Part model, mm, in its own coordinate system. A direction names the side the tool comes from. Give positions to 0.01 mm unless a question says otherwise; leave off trailing zeros. Loops run counter-clockwise (first coordinate to the right, second up) from the corner with the lowest first, then second, coordinate; pieces in that order, holes last. Notation, with made-up numbers: M 55,-34 L 69,-34 A31 ccw 69,5 Z; hole C 1.25,76 d7. An arc over 180 degrees is marked long. Answer in a Markdown table with one row per item.
from build123d import *

# Parameters (mm, degrees)
ESQUISSE1_W              = 130
ESQUISSE1_H              = 167
BOSS_EXTRU_1_DEPTH       = 3
ESQUISSE6_R              = 3.5
ESQUISSE6_R_2            = 4
BOSS_EXTRU_3_DEPTH       = 5
ESQUISSE11_W             = 67
ESQUISSE11_H             = 10
BOSS_EXTRU_6_DEPTH       = 49
ENL_V_MAT_EXTRU_3_REACH  = 113.374
ESQUISSE12_R             = 7.5
ESQUISSE12_W             = 7
ESQUISSE12_H             = 10
ESQUISSE13_R             = 9.4
ENL_V_MAT_EXTRU_4_DEPTH  = 65.5
BOSS_EXTRU_7_DEPTH       = 1.5
ESQUISSE15_W             = 20
ESQUISSE15_H             = 4
ENL_V_MAT_EXTRU_5_DEPTH  = 43.7
ESQUISSE16_W             = 21
ESQUISSE16_H             = 10
BOSS_EXTRU_8_DEPTH       = 78.5
ESQUISSE17_W             = 10.5
ESQUISSE17_H             = 10
ESQUISSE17_W_2           = 20
ESQUISSE17_H_2           = 4
ENL_V_MAT_EXTRU_6_DEPTH  = 24.2
ENL_V_MAT_EXTRU_7_REACH  = 148.361
ESQUISSE18_R             = 7.5
ESQUISSE19_R             = 9.4
ENL_V_MAT_EXTRU_8_DEPTH  = 65.5
BOSS_EXTRU_9_DEPTH       = 1.5
ESQUISSE21_R             = 2.3
ESQUISSE21_R_2           = 1.8
ENL_V_MAT_EXTRU_9_DEPTH  = 6.1
ESQUISSE22_R             = 1.7
ENL_V_MAT_EXTRU_10_DEPTH = 107.288522428


with BuildPart() as part:
    # Esquisse1 → Boss.-Extru.1 (new body)
    with BuildSketch(Plane(origin=(0, 0, 0), x_dir=(1, 0, 0), z_dir=(0, 1, 0))):
        Rectangle(ESQUISSE1_W, ESQUISSE1_H)
    extrude(amount=BOSS_EXTRU_1_DEPTH)

    # Esquisse6 → Boss.-Extru.3 (add)
    with BuildSketch(Plane(origin=(0, 3, 0), x_dir=(1, 0, 0), z_dir=(0, 1, 0))):
        with Locations(Location((-8, -73.5, 0), (0, 0, 90))):
            Circle(ESQUISSE6_R)
        with Locations(Location((-8, -50.5, 0), (0, 0, 90))):
            Circle(ESQUISSE6_R)
        with Locations(Location((50, -50.5, 0), (0, 0, 90))):
            Circle(ESQUISSE6_R)
        with Locations(Location((50, -73.5, 0), (0, 0, 90))):
            Circle(ESQUISSE6_R)
        with Locations(Location((56, 43.5, 0), (0, 0, 90))):
            Circle(ESQUISSE6_R_2)
        with Locations(Location((56, -34.732, 0), (0, 0, 90))):
            Circle(ESQUISSE6_R_2)
        with Locations(Location((-3.436, -35.232, 0), (0, 0, 90))):
            Circle(ESQUISSE6_R_2)
    extrude(amount=BOSS_EXTRU_3_DEPTH)

    # Esquisse11 → Boss.-Extru.6 (add)
    with BuildSketch(Plane.ZY.offset(65)):
        with Locations((-27.5, 8)):
            Rectangle(ESQUISSE11_W, ESQUISSE11_H)
    extrude(amount=-BOSS_EXTRU_6_DEPTH)

    # Esquisse12 → Enlèv. mat.-Extru.3 (cut, up to next)
    with BuildSketch(Plane.XY.offset(6), mode=Mode.PRIVATE) as enl_v_mat_extru_3_sk1:
        with Locations((-47.2, 13)):
            Circle(ESQUISSE12_R)
    enl_v_mat_extru_3_tool1 = extrude(enl_v_mat_extru_3_sk1.sketch, amount=-ENL_V_MAT_EXTRU_3_REACH, mode=Mode.PRIVATE) & part.part
    # Esquisse12 → Enlèv. mat.-Extru.3 (cut, up to next)
    with BuildSketch(Plane.XY.offset(6), mode=Mode.PRIVATE) as enl_v_mat_extru_3_sk2:
        with Locations((-26.8, 13)):
            Circle(ESQUISSE12_R)
    enl_v_mat_extru_3_tool2 = extrude(enl_v_mat_extru_3_sk2.sketch, amount=-ENL_V_MAT_EXTRU_3_REACH, mode=Mode.PRIVATE) & part.part
    # Esquisse12 → Enlèv. mat.-Extru.3 (cut, up to next)
    with BuildSketch(Plane.XY.offset(6), mode=Mode.PRIVATE) as enl_v_mat_extru_3_sk3:
        with Locations((-61.5, 8)):
            Rectangle(ESQUISSE12_W, ESQUISSE12_H)
    enl_v_mat_extru_3_tool3 = extrude(enl_v_mat_extru_3_sk3.sketch, amount=-ENL_V_MAT_EXTRU_3_REACH, mode=Mode.PRIVATE) & part.part
    add(enl_v_mat_extru_3_tool1.solids().sort_by_distance((-47.2, 13, 6))[0], mode=Mode.SUBTRACT)
    add(enl_v_mat_extru_3_tool2.solids().sort_by_distance((-26.8, 13, 6))[0], mode=Mode.SUBTRACT)
    add(enl_v_mat_extru_3_tool3.solids().sort_by_distance((-61.5, 8, 6))[0], mode=Mode.SUBTRACT)

    # Esquisse13 → Enlèv. mat.-Extru.4 (cut)
    with BuildSketch(Plane.XY.offset(6)):
        with Locations((-47.2, 13)):
            Circle(ESQUISSE13_R)
        with Locations((-26.8, 13)):
            Circle(ESQUISSE13_R)
    extrude(amount=-ENL_V_MAT_EXTRU_4_DEPTH, mode=Mode.SUBTRACT)

    # Esquisse14 → Boss.-Extru.7 (add)
    with BuildSketch(Plane.XY.offset(6)):
        with BuildLine():
            Line((-58, 13), (-54.7, 13))
            ThreePointArc((-54.7, 13), (-47.2, 5.5), (-39.7, 13))
            Line((-39.7, 13), (-34.3, 13))
            ThreePointArc((-34.3, 13), (-26.8, 5.5), (-19.3, 13))
            Line((-19.3, 13), (-16, 13))
            Line((-16, 13), (-16, 3))
            Line((-16, 3), (-58, 3))
            Line((-58, 3), (-58, 13))
        make_face()
    extrude(amount=-BOSS_EXTRU_7_DEPTH)

    # Esquisse15 → Enlèv. mat.-Extru.5 (cut)
    with BuildSketch(Plane.ZY.offset(58)):
        with Locations((-28, 11)):
            Rectangle(ESQUISSE15_W, ESQUISSE15_H)
    extrude(amount=-ENL_V_MAT_EXTRU_5_DEPTH, mode=Mode.SUBTRACT)

    # Esquisse16 → Boss.-Extru.8 (add)
    with BuildSketch(Plane(origin=(65, 0, 0), x_dir=(0, 0, -1), z_dir=(1, 0, 0))):
        with Locations((69.6, 8)):
            Rectangle(ESQUISSE16_W, ESQUISSE16_H)
    extrude(amount=-BOSS_EXTRU_8_DEPTH)

    # Esquisse17 → Enlèv. mat.-Extru.6 (cut)
    with BuildSketch(Plane(origin=(0, 0, -80.1), x_dir=(-1, 0, 0), z_dir=(0, 0, -1))):
        with Locations((-59.75, 8)):
            Rectangle(ESQUISSE17_W, ESQUISSE17_H)
        with Locations((-20.5, 11)):
            Rectangle(ESQUISSE17_W_2, ESQUISSE17_H_2)
    extrude(amount=-ENL_V_MAT_EXTRU_6_DEPTH, mode=Mode.SUBTRACT)

    # Esquisse18 → Enlèv. mat.-Extru.7 (cut, up to next)
    with BuildSketch(Plane(origin=(54.5, 0, 0), x_dir=(0, 0, -1), z_dir=(1, 0, 0)), mode=Mode.PRIVATE) as enl_v_mat_extru_7_sk1:
        with Locations((69.6, 13)):
            Circle(ESQUISSE18_R)
    enl_v_mat_extru_7_tool1 = extrude(enl_v_mat_extru_7_sk1.sketch, amount=-ENL_V_MAT_EXTRU_7_REACH, mode=Mode.PRIVATE) & part.part
    add(enl_v_mat_extru_7_tool1.solids().sort_by_distance((54.5, 13, -69.6))[0], mode=Mode.SUBTRACT)

    # Esquisse19 → Enlèv. mat.-Extru.8 (cut)
    with BuildSketch(Plane(origin=(54.5, 0, 0), x_dir=(0, 0, -1), z_dir=(1, 0, 0))):
        with Locations((69.6, 13)):
            Circle(ESQUISSE19_R)
    extrude(amount=-ENL_V_MAT_EXTRU_8_DEPTH, mode=Mode.SUBTRACT)

    # Esquisse20 → Boss.-Extru.9 (add)
    with BuildSketch(Plane(origin=(54.5, 0, 0), x_dir=(0, 0, -1), z_dir=(1, 0, 0))):
        with BuildLine():
            Line((59.1, 13), (62.1, 13))
            ThreePointArc((62.1, 13), (69.6, 5.5), (77.1, 13))
            Line((77.1, 13), (80.1, 13))
            Line((80.1, 13), (80.1, 3))
            Line((80.1, 3), (59.1, 3))
            Line((59.1, 3), (59.1, 13))
        make_face()
    extrude(amount=-BOSS_EXTRU_9_DEPTH)

    # Esquisse21 → Enlèv. mat.-Extru.9 (cut)
    with BuildSketch(Plane(origin=(0, 8, 0), x_dir=(1, 0, 0), z_dir=(0, 1, 0))):
        with Locations(Location((56, 43.5, 0), (0, 0, 270))):
            Circle(ESQUISSE21_R)
        with Locations(Location((56, -34.732, 0), (0, 0, 270))):
            Circle(ESQUISSE21_R)
        with Locations(Location((-3.436, -35.232, 0), (0, 0, 270))):
            Circle(ESQUISSE21_R)
        with Locations(Location((50, -50.5, 0), (0, 0, 270))):
            Circle(ESQUISSE21_R_2)
        with Locations(Location((50, -73.5, 0), (0, 0, 270))):
            Circle(ESQUISSE21_R_2)
        with Locations(Location((-8, -50.5, 0), (0, 0, 270))):
            Circle(ESQUISSE21_R_2)
        with Locations(Location((-8, -73.5, 0), (0, 0, 270))):
            Circle(ESQUISSE21_R_2)
    extrude(amount=-ENL_V_MAT_EXTRU_9_DEPTH, mode=Mode.SUBTRACT)

    # Esquisse22 → Enlèv. mat.-Extru.10 (cut, through all)
    with BuildSketch(Plane(origin=(0, 3, 0), x_dir=(1, 0, 0), z_dir=(0, 1, 0))):
        with Locations(Location((-60, 71.5, 0), (0, 0, 270))):
            Circle(ESQUISSE22_R)
        with Locations(Location((60, 71.5, 0), (0, 0, 270))):
            Circle(ESQUISSE22_R)
        with Locations(Location((60, -58.5, 0), (0, 0, 270))):
            Circle(ESQUISSE22_R)
        with Locations(Location((-60, -58.5, 0), (0, 0, 270))):
            Circle(ESQUISSE22_R)
    extrude(amount=-ENL_V_MAT_EXTRU_10_DEPTH, mode=Mode.SUBTRACT)


solid = part.part
(1) Saw through at A-A (z = 58.5). Write the cut outline in (x, y), plus the area to 3 significant figures.
Recorded:
| item | result |
|---|---|
| outline | M -65,0 L -61.7,0 L -61.7,3 L -65,3 Z; M -58.3,0 L 58.3,0 L 58.3,3 L -58.3,3 Z; M 61.7,0 L 65,0 L 65,3 L 61.7,3 Z |
| area | 370 mm^2 |
(2) Saw through at B-B (x = 50). Write the cut outline in (y, z).
Recorded:
| item | result |
|---|---|
| outline | M 0,-83.5 L 3,-83.5 L 3,-80.1 L 13,-80.1 L 13,-79 A9.4 cw 13,-60.2 L 13,-59.1 L 3,-59.1 L 3,47 L 8,47 L 8,48.7 L 1.9,48.7 L 1.9,52.3 L 8,52.3 L 8,54 L 3,54 L 3,70 L 8,70 L 8,71.7 L 1.9,71.7 L 1.9,75.3 L 8,75.3 L 8,77 L 3,77 L 3,83.5 L 0,83.5 Z |
(3) Drill centre lines: line 1 along X through (y, z) = (5.75, 73.5); line 2 along X through (y, z) = (1.25, -71.5); line 3 along Z through (x, y) = (-21.5, 7). Where is each one in solid material? Low to high.
Recorded:
| item | result |
|---|---|
| line 1 | x = -11.5 to -9.8, -6.2 to -4.5, 46.5 to 48.2, 51.8 to 53.5 |
| line 2 | x = -65 to -61.7, -58.3 to 58.3, 61.7 to 65 |
| line 3 | z = -61 to -59.5, 4.5 to 6 |
(4) Pull direction Z, two halves, no side cores. Call faces 1 (the face through (-37, 11, -38)), 2 (the face through (58, 8, 33)), 3 (the face through (21, 8, -80.1)): +Z half, -Z half, draft (parallel to the pull), parting line (faces both ways), or undercut.
Recorded:
| item | result |
|---|---|
| face 1 | undercut |
| face 2 | draft |
| face 3 | -Z half |
(5) Saw through at C-C (z = -71.5). Write the cut outline in (x, y).
Recorded:
| item | result |
|---|---|
| outline | M -65,0 L -61.7,0 L -61.7,3 L -65,3 Z; M -58.3,0 L 58.3,0 L 58.3,3 L 54.5,3 L 54.5,5.74 L 53,5.74 L 53,3.79 L -11,3.79 L -11,5.74 L -13.5,5.74 L -13.5,3 L -58.3,3 Z; M 61.7,0 L 65,0 L 65,3 L 61.7,3 Z |
(6) Which spindle directions (+Z, -Z, +X, -X, +Y, -Y) get a long thin tool onto all of the face, cutting with end or side? Do faces 4 (the face through (58, 8, -45)), 5 (the face through (-13.5, 5, -69)), 6 (the face through (21, 8, -59.1)), 7 (the face through (53.755, 4.993, 34.233)). Say none if no direction does.
Recorded:
| item | result |
|---|---|
| face 4 | +Z, +X, +Y |
| face 5 | +Z, -Z, +Y |
| face 6 | +X, +Y |
| face 7 | +Y |
(7) Pin check, flat tips, straight feed: pin 1 Ø4 at (x, y) = (-8, 7) entering from +Z; pin 2 Ø5 at (x, z) = (41, 10) entering from +Y; pin 3 Ø2.5 at (x, z) = (-3, 35) entering from +Y; pin 4 Ø3 at (x, z) = (50, 73.5) entering from -Y. Stop position of each tip, or through.
Recorded:
| item | result |
|---|---|
| pin 1 | stops at z = 77 |
| pin 2 | stops at y = 3 |
| pin 3 | stops at y = 1.9 |
| pin 4 | stops at y = 0 |
(8) Saw through at D-D (x = -21.5). Write the cut outline in (y, z).
Recorded:
| item | result |
|---|---|
| outline | M 0,-83.5 L 3,-83.5 L 3,-61 L 7.69,-61 L 7.69,-59.5 L 5.24,-59.5 L 5.24,4.5 L 7.69,4.5 L 7.69,6 L 3,6 L 3,83.5 L 0,83.5 Z |
